Geometry check sheet. Reference: drawing and pictorial views, mm from the part's lowest x, y, z. A direction names the side the tool comes from. Give positions to 0.01 mm unless a question says otherwise; leave off trailing zeros. Loops run counter-clockwise (first coordinate to the right, second up) from the corner with the lowest first, then second, coordinate; pieces in that order, holes last. Notation, with made-up numbers: (18.25, 29.25) -> (61.25, 29.25) arc R22 cw to (61.25, 64.25) -> close; hole circle Ø6 at (63.25, 36). An arc over 180 degrees is marked (long way). Write each question's results on one line, items separated by ' | '. Start each with the question number.
1. Material ranges on L1, parallel to X at y = 4.5, z = 13; L2, parallel to X at y = 4.5, z = 17.75, recorded low to high. Write a range as from..to.
2. Mould release check, pull along Y, two halves, no side actions. Record for the marked faces 3, 4 and 5: +Y half, -Y half, draft (parallel to the pull), parting line (faces both ways), or undercut.
3. Tool access check on the marked faces 1 and 2. Record the directions out of +Z, -Z, +X, -X, +Y, -Y that give a thin tool (end or side, any length) a straight path to the whole face; none if there is none.
4. Cross-section at D-D on z = 2.25. Record the boundary of the cut face in (x, y), and give its area (3 significant figures).
5. Gauge pin test, flat ends, axial feed: pin 1 Ø3 at (y, z) = (2.5, 13.5) entering from +X; pin 2 Ø2 at (y, z) = (1, 3) entering from +X; pin 3 Ø5 at (y, z) = (8, 18.5) entering from +X. Record the tip position at first contact, or that the pin passes through.
6. Cross-section at B-B on z = 7. Record the boundary of the cut face in (x, y).
7. Cross-section at A-A on y = 4.55. Record the boundary of the cut face in (x, z), and give its area (3 significant figures).
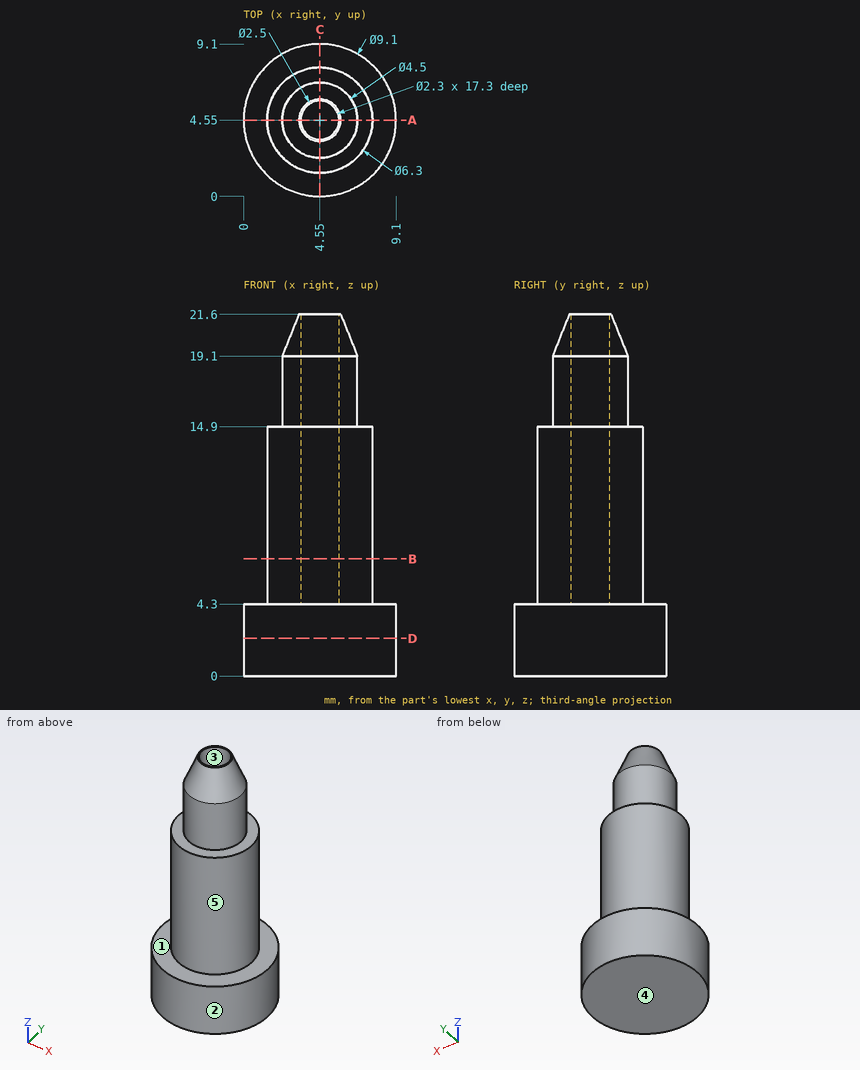
Geometry says:
1) L1: 1.4..3.4, 5.7..7.7 | L2: 2.3..3.4, 5.7..6.8
2) face 3: undercut | face 4: draft | face 5: parting line
3) face 1: +Z | face 2: +Z, -Z
4) outline: circle Ø9.1 at (4.55, 4.55) | area: 65.0 mm^2
5) pin 1: x = 7.65 | pin 2: x = 8.32 | pin 3: x = 6.59
6) outline: circle Ø6.3 at (4.55, 4.55); hole circle Ø2.3 at (4.55, 4.55)
7) outline: (0, 0) -> (9.1, 0) -> (9.1, 4.3) -> (7.7, 4.3) -> (7.7, 14.9) -> (6.8, 14.9) -> (6.8, 19.1) -> (5.8, 21.6) -> (5.7, 21.6) -> (5.7, 4.3) -> (3.4, 4.3) -> (3.4, 21.6) -> (3.3, 21.6) -> (2.3, 19.1) -> (2.3, 14.9) -> (1.4, 14.9) -> (1.4, 4.3) -> (0, 4.3) -> close | area: 93.8 mm^2
